Can you work these out from the model? Positions are in its coordinate system, mm. Face numbers are marked on the shaded views. A direction names the side the tool comes from. Give positions to 0.01 mm unless a question says otherwise; leave off trailing zeros. Order: outer loops, then holes, each group sorted by start corner. A loop starts at its lowest first (then second) coordinate and runs counter-clockwise, first axis right, second up. Notation, with made-up numbers: (88, -0.75) -> (93, -0.75) arc R22 ccw to (93, 10.25) -> close; hole circle Ø8 at (87, -8.5). An arc over 180 degrees is marked (long way). Answer as a JSON object with one key per item and string values.
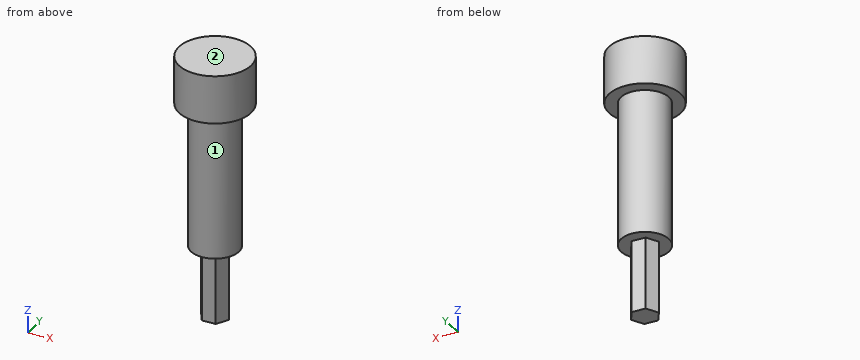
Autodesk Inventor part; units mm, degrees
ref_plane "YZ Plane" through (0, 0, 0) normal (1, 0, 0) x (0, 1, 0)
ref_plane "XZ Plane" through (0, 0, 0) normal (0, 1, 0) x (-1, 0, 0)
ref_plane "XY Plane" through (0, 0, 0) normal (0, 0, 1) x (1, 0, 0)
sketch "Sketch1" plane through (0, 0, 0) normal (0, 0, 1) x (1, 0, 0)
  circle A0 centre (0, 0) radius 19.05
  dimension "d0" = 38.1
extrude "Extrusion1" add sketch "Sketch1" against normal blind 25.4
sketch "Sketch3" plane through (0, 0, -25.4) normal (0, 0, -1) x (-1, 0, 0)
  circle A0 centre (0, 0) radius 12.7
  dimension "d4" = 25.4
extrude "Extrusion2" add sketch "Sketch3" along normal blind 76.2
sketch "Sketch4" plane through (0, 0, -101.6) normal (0, 0, -1) x (-1, 0, 0)
  line L0 (-3.6662, -6.35) -> (-7.3323, 0)
  line L1 (-7.3323, 0) -> (-3.6662, 6.35)
  line L2 (-3.6662, 6.35) -> (3.6662, 6.35)
  line L3 (3.6662, 6.35) -> (7.3323, 0)
  line L4 (7.3323, 0) -> (3.6662, -6.35)
  line L5 (3.6662, -6.35) -> (-3.6662, -6.35)
  point P0 (0, 0)
  point P1 (0, 0)
  dimension "d7" = 12.7
extrude "Extrusion3" add sketch "Sketch4" along normal blind 38.1
properties part number "ForTurningForkDrive"
1. Will these pins go through, and if not, where does the flat tip stop? pin 1 Ø3 at (y, z) = (3, -97) entering from +X; pin 2 Ø8 at (y, z) = (-12.5, -62) entering from +X; pin 3 Ø2 at (x, z) = (0, -115) entering from -Y.
Worked answers:
{"pin 1": "x = 12.61", "pin 2": "x = 9.44", "pin 3": "y = -6.35"}
2. If we section it at B-B on y = 11: Please give me the cut outline in (x, z).
Worked answers:
{"outline": "(-15.55, -25.4) -> (-6.35, -25.4) -> (-6.35, -101.6) -> (6.35, -101.6) -> (6.35, -25.4) -> (15.55, -25.4) -> (15.55, 0) -> (-15.55, 0) -> close"}
3. For the marked faces 1 and 2, which set-ups out of +Z, -Z, +X, -X, +Y, -Y let a thin tool reach every point of the face, with its end or its side?
Worked answers:
{"face 1": "-Z", "face 2": "+Z, +X, -X, +Y, -Y"}
4. If we section it at A-A on x = 0: Please give me the cut outline in (y, z).
Worked answers:
{"outline": "(-19.05, -25.4) -> (-12.7, -25.4) -> (-12.7, -101.6) -> (-6.35, -101.6) -> (-6.35, -139.7) -> (6.35, -139.7) -> (6.35, -101.6) -> (12.7, -101.6) -> (12.7, -25.4) -> (19.05, -25.4) -> (19.05, 0) -> (-19.05, 0) -> close"}
5. Please list where these lines run through material, in increasing order: L1, parallel to Z at x = -2, y = -14; L2, parallel to Z at x = -10.5, y = -0.5; L3, parallel to Y at x = -6.5, z = -119.
Worked answers:
{"L1": "-25.4 to 0", "L2": "-101.6 to 0", "L3": "-1.44 to 1.44"}
6. If we section it at D-D on y = 5: Please give me the cut outline in (x, z), then the cut area to 3 significant figures.
Worked answers:
{"outline": "(-18.38, -25.4) -> (-11.67, -25.4) -> (-11.67, -101.6) -> (-4.45, -101.6) -> (-4.45, -139.7) -> (4.45, -139.7) -> (4.45, -101.6) -> (11.67, -101.6) -> (11.67, -25.4) -> (18.38, -25.4) -> (18.38, 0) -> (-18.38, 0) -> close", "area": "3,050 mm²"}
7. If we section it at C-C on z = -121: Please give me the cut outline in (x, y).
Worked answers:
{"outline": "(-7.33, 0) -> (-3.67, -6.35) -> (3.67, -6.35) -> (7.33, 0) -> (3.67, 6.35) -> (-3.67, 6.35) -> close"}
